Input: dimensioned drawing with shaded views. Units: mm. Origin: part minimum x, y, z. A direction names the side the tool comes from. Give positions to 0.01 mm unless a question says otherwise; leave off trailing zeros. Loops run counter-clockwise (first coordinate to the right, second up) from the corner with the lowest first, then second, coordinate; pieces in that order, holes last. Notation, with made-up numbers: (86.25, -4) -> (107.25, -4) arc R17 ccw to (107.25, 23) -> close; hole circle Ø2 at (45, 68). An arc over 180 degrees is marked (long way). One line per question, with ' | ' between items. Start each with the question number.
Item 1: Section B-B on y = 148. Return loops of the section in (x, z).
Item 2: Section C-C on z = 27.5. Return loops of the section in (x, y), then the cut area to 3 significant figures.
Item 3: Mould query, pull axis Z, two halves, no side actions, for the marked faces 1, 2, 3 and 4. Classes: released by +Z, released by -Z, zero draft, split by the parting line, or undercut.
Item 4: Set-up query: the marked faces 5 and 6. Return all of +Z, -Z, +X, -X, +Y, -Y with unobstructed straight access to the full face (end or side cutting, diameter ignored); none if empty.
Item 5: Section A-A on x = 35. Return loops of the section in (y, z), then the cut area to 3 significant figures.
Item 6: Section D-D on z = 48. Return loops of the section in (x, y), then the cut area to 3 significant figures.
Item 7: Material intervals for line 1 along X through (y, z) = (113.5, 40); line 2 along X through (y, z) = (158, 47), sorted ascending. Write a range as [from, to].
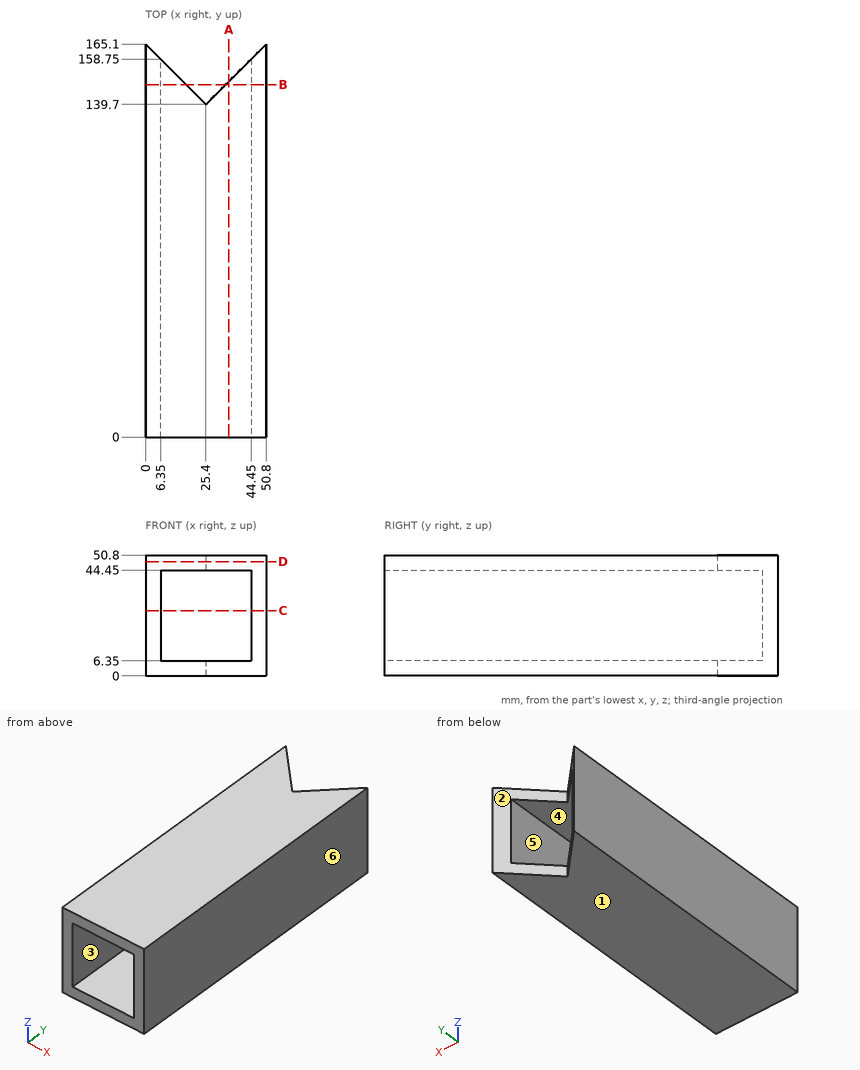
Result sheet:
1) outline: (0, 0) -> (17.1, 0) -> (17.1, 6.35) -> (6.35, 6.35) -> (6.35, 44.45) -> (17.1, 44.45) -> (17.1, 50.8) -> (0, 50.8) -> close; (33.7, 0) -> (50.8, 0) -> (50.8, 50.8) -> (33.7, 50.8) -> (33.7, 44.45) -> (44.45, 44.45) -> (44.45, 6.35) -> (33.7, 6.35) -> close
2) outline: (0, 0) -> (6.35, 0) -> (6.35, 158.75) -> (0, 165.1) -> close; (44.45, 0) -> (50.8, 0) -> (50.8, 165.1) -> (44.45, 158.75) -> close | area: 2,060 mm²
3) face 1: released by -Z | face 2: zero draft | face 3: undercut | face 4: undercut
4) face 5: +Y, -Y | face 6: +Z, -Z, +X, +Y, -Y
5) outline: (0, 0) -> (149.3, 0) -> (149.3, 6.35) -> (0, 6.35) -> close; (0, 44.45) -> (149.3, 44.45) -> (149.3, 50.8) -> (0, 50.8) -> close | area: 1,900 mm²
6) outline: (0, 0) -> (50.8, 0) -> (50.8, 165.1) -> (25.4, 139.7) -> (0, 165.1) -> close | area: 7,740 mm²
7) line 1: x = [0, 6.35], [44.45, 50.8] | line 2: x = [0, 7.1], [43.7, 50.8]
